Could you check a few things on this drawing? It's one solid part, dimensions in mm from its lowest x, y, z. A direction names the side the tool comes from. Round coordinates to 2 decimals unless told otherwise and drop trailing zeros. Write each loop counter-clockwise with the first axis right and the second up, starting at its lowest first coordinate (ties: lowest second). Pieces come first, ordered by that corner, then holes. Notation, with made-up numbers: (-25, 61) -> (26, 61) arc R23 ccw to (26, 90) -> close; hole circle Ø9 at (23, 87.5). An arc over 180 degrees is marked (long way). Answer in a Markdown table with one row per item. Add a question column.
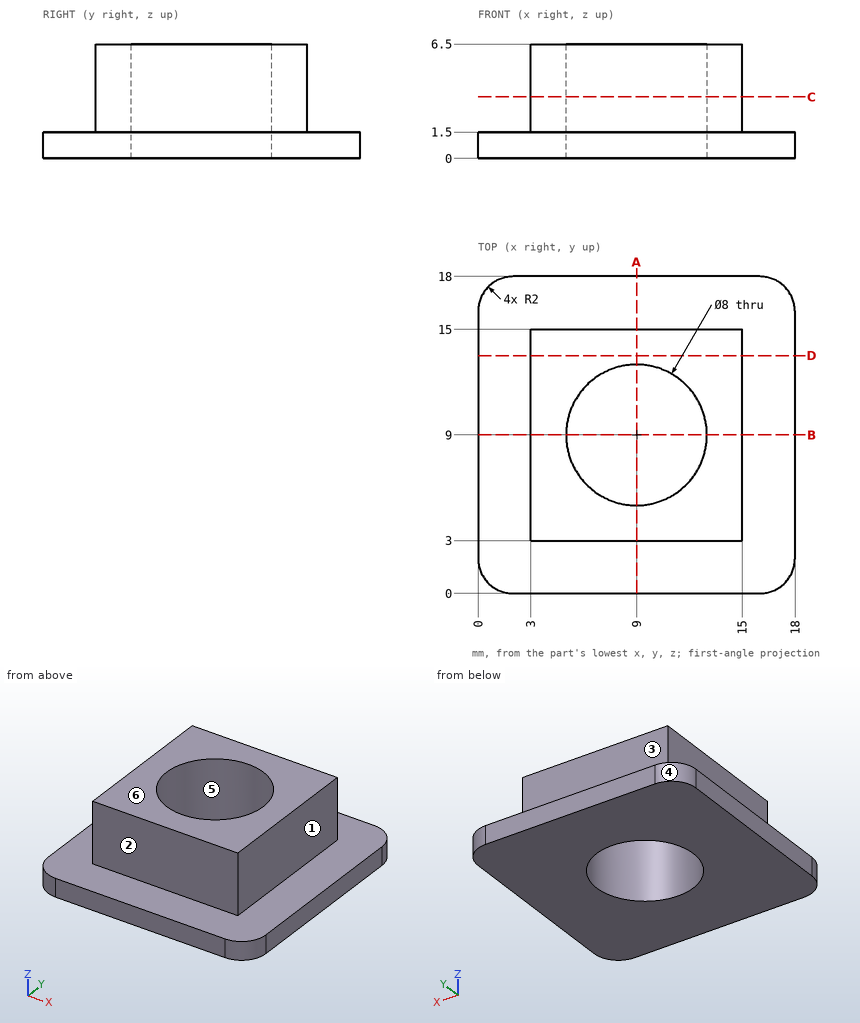
(1) Suppose I cut it at C-C, the plane z = 3.5. Please give me the cut outline in (x, y), then the cut area to 3 significant figures.
(2) Suppose I cut it at A-A, the plane x = 9. Please give me the cut outline in (y, z).
(3) For P1, Ø1, axis at x = 8.5, z = 5.5, coming from the -Y side; P2, Ø2.5, axis at x = 10.5, z = 4.5, coming from the +Y side; P3, Ø1.5, axis at x = 8.5, y = 2, coming from the +Z side, each with a flat end and sliding along its axis, tell me the tip position at first contact or that it passes through.
(4) I need wall thicknesses on L1, parallel to Y at x = 9, z = 3.25; L2, parallel to Z at x = 16.5, y = 17.25; L3, parallel to Y at x = 14.75, z = 2. Which ranges of each line are inside material? Lowest first, please.
(5) If we mould it in two halves opening along X, with no side actions, what happens to the marked faces 4, 5 and 6? For each: pulls with the +X half, pulls with the -X half, needs draft (parallel to the pull), parting line crosses it, or undercut.
(6) Suppose I cut it at D-D, the plane y = 13.5. Please give me the cut outline in (x, z).
(7) On a 3-axis mill with a long thin cutter (end or side, diameter ignored), from which of +Z, -Z, +X, -X, +Y, -Y can I reach the whole of each face in a straight line? I mean the marked faces 1, 2 and 3. Say none if no direction works.
Response:
| question | item | result |
|---|---|---|
| 1 | outline | (3, 3) -> (15, 3) -> (15, 15) -> (3, 15) -> close; hole circle Ø8 at (9, 9) |
| 1 | area | 93.7 mm² |
| 2 | outline | (0, 0) -> (5, 0) -> (5, 6.5) -> (3, 6.5) -> (3, 1.5) -> (0, 1.5) -> close; (13, 0) -> (18, 0) -> (18, 1.5) -> (15, 1.5) -> (15, 6.5) -> (13, 6.5) -> close |
| 3 | P1 | y = 3 |
| 3 | P2 | y = 15 |
| 3 | P3 | z = 1.5 |
| 4 | L1 | 3 to 5, 13 to 15 |
| 4 | L2 | 0 to 1.5 |
| 4 | L3 | 3 to 15 |
| 5 | face 4 | pulls with the -X half |
| 5 | face 5 | undercut |
| 5 | face 6 | needs draft |
| 6 | outline | (0, 0) -> (18, 0) -> (18, 1.5) -> (15, 1.5) -> (15, 6.5) -> (3, 6.5) -> (3, 1.5) -> (0, 1.5) -> close |
| 7 | face 1 | +Z, +X, +Y, -Y |
| 7 | face 2 | +Z, +X, -X, -Y |
| 7 | face 3 | +Z, +X, -X, +Y |
